from build123d import *

# Parameters (mm, degrees)
PAD_DEPTH    = 1
PAD001_DEPTH = 3


with BuildPart() as part:
    # Sketch → Pad (new body)
    with BuildSketch(Plane.XY):
        with BuildLine():
            Line((4, 0), (95, 0))
            Line((95, 110), (95, 0))
            Line((95, 110), (4, 110))
            ThreePointArc((4, 110), (1.171573, 108.828427), (0, 106))
            Line((0, 106), (0, 4))
            ThreePointArc((0, 4), (1.171573, 1.171573), (4, 0))
        make_face()
    extrude(amount=PAD_DEPTH)

    # Sketch001 → Pad001 (new body)
    with BuildSketch(Plane.XY.offset(1)):
        with BuildLine():
            Line((4, 0), (95, 0))
            Line((95, 0), (95, 0.9))
            Line((95, 0.9), (3.9, 0.9))
            ThreePointArc((0.9, 3.9), (1.77868, 1.77868), (3.9, 0.9))
            Line((0.9, 3.9), (0.9, 106.1))
            ThreePointArc((3.9, 109.1), (1.77868, 108.22132), (0.9, 106.1))
            Line((3.9, 109.1), (95, 109.1))
            Line((95, 109.1), (95, 110))
            Line((95, 110), (4, 110))
            ThreePointArc((4, 110), (1.171573, 108.828427), (0, 106))
            Line((0, 106), (0, 4))
            ThreePointArc((0, 4), (1.171573, 1.171573), (4, 0))
        make_face()
    extrude(amount=PAD001_DEPTH)


solid = part.part
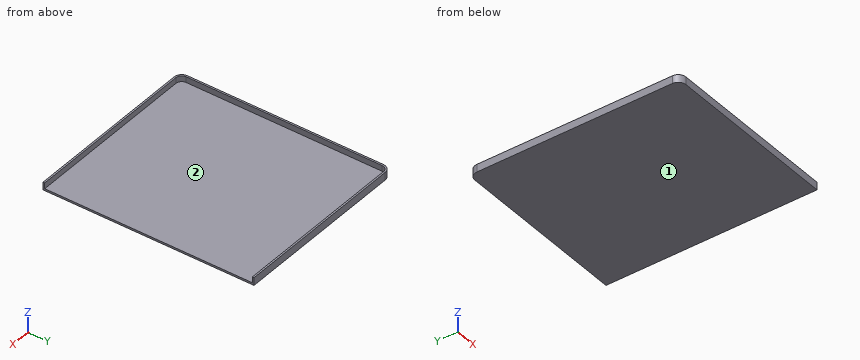
Design review of the part built by this model. Coordinates are the model's own, in mm. Face numbers are marked on the shaded views. Round coordinates to 2 decimals unless told otherwise and drop trailing zeros. Write each loop counter-clockwise with the first axis right and the second up, starting at its lowest first coordinate (ties: lowest second). Pieces come first, ordered by that corner, then holes. Notation, with made-up numbers: (-6, 27) - (17, 27) arc R13 ccw to (17, 42) - close; hole circle Ø8 at (38.5, 89). An arc over 180 degrees is marked (long way). Use a Markdown table: item, result. Add a question column.
1. Wall thickness on probe 1 along Y at (x, z) = (86, 1.05); probe 2 along X at (y, z) = (26.5, 2.95); probe 3 along Z at (x, y) = (67, 21.5): over which ranges is each line inside the solid? List them lowest first.
2. Mouldability with a two-part tool opening along Y and no side actions: class the marked faces 1 and 2 as +Y half, -Y half, draft (parallel to the pull), parting line (faces both ways), or undercut.
3. We need section A-A (y = 77.5). State the section outline as (x, z) points, then the cut area to 3 significant figures.
4. We need section C-C (x = 61). State the section outline as (y, z) points.
5. Clearance check with flat-ended pins moving along their axes: pin 1 (8 mm diameter, centred on x = 80.5, y = 65, fed in from +Z); pin 2 (1 mm diameter, centred on x = 30, y = 15, fed in from -Z). State where each tip first meets the part, or that it passes through.
6. We need section B-B (z = 2.4). State the section outline as (x, y) points, then the cut area to 3 significant figures.
Output:
| question | item | result |
|---|---|---|
| 1 | probe 1 | y = 0 to 0.9, 109.1 to 110 |
| 1 | probe 2 | x = 0 to 0.9 |
| 1 | probe 3 | z = 0 to 1 |
| 2 | face 1 | draft |
| 2 | face 2 | undercut |
| 3 | outline | (0, 0) - (95, 0) - (95, 1) - (0.9, 1) - (0.9, 4) - (0, 4) - close |
| 3 | area | 97.7 mm2 |
| 4 | outline | (0, 0) - (110, 0) - (110, 4) - (109.1, 4) - (109.1, 1) - (0.9, 1) - (0.9, 4) - (0, 4) - close |
| 5 | pin 1 | stops at z = 1 |
| 5 | pin 2 | stops at z = 0 |
| 6 | outline | (0, 4) arc R4 ccw to (4, 0) - (95, 0) - (95, 0.9) - (3.9, 0.9) arc R3 cw to (0.9, 3.9) - (0.9, 106.1) arc R3 cw to (3.9, 109.1) - (95, 109.1) - (95, 110) - (4, 110) arc R4 ccw to (0, 106) - close |
| 6 | area | 265 mm2 |
